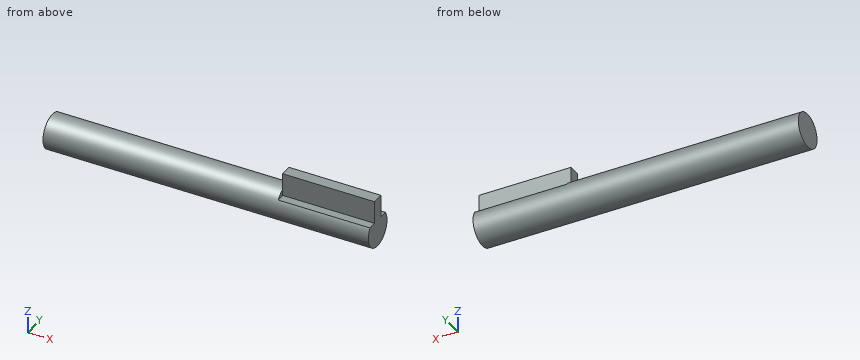
from build123d import *

# Parameters (mm, degrees)
F0_R     = 9.525
F1_DEPTH = 179.9844
F3_DEPTH = 50.8
F4_W     = 50.8
F4_H     = 6.35
F5_DEPTH = 12.7


with BuildPart() as f1:
    # F0 (on Right) → F1 (new body)
    with BuildSketch(Plane.YZ):
        Circle(F0_R)
    extrude(amount=-F1_DEPTH)

    # F2 (on face) → F3 (cut)
    with BuildSketch(Plane.YZ):
        with BuildLine():
            Line((-7.7629294276, 5.5192890577), (0, 5.5192890577))
            Line((0, 5.5192890577), (7.7629294276, 5.5192890577))
            ThreePointArc((7.7629294276, 5.5192890577), (0, 9.525), (-7.7629294276, 5.5192890577))
        make_face()
    extrude(amount=-F3_DEPTH, mode=Mode.SUBTRACT)

    # F4 (on face) → F5 (join)
    with BuildSketch(Plane.XY.offset(5.5192890577)):
        with Locations((-25.4, 0)):
            Rectangle(F4_W, F4_H)
    extrude(amount=F5_DEPTH)


solid = f1.part
Geometry check sheet. Reference: the model listing, model coordinates, mm. Give positions to 0.01 mm unless a question says otherwise; leave off trailing zeros. Loops run counter-clockwise (first coordinate to the right, second up) from the corner with the lowest first, then second, coordinate; pieces in that order, holes last. Notation, with made-up numbers: M 5.25,21.25 L 53.25,21.25 A24 cw 53.25,59.25 Z; hole C 30.25,58.25 d3. An arc over 180 degrees is marked long. Write each question's results on one line, items separated by ' | '.
1) Section check B-B, the plane z = 7. Record the boundary of the cut face in (x, y) (3 decimals), plus the area to 3 significant figures.
Answers follow:
outline: M -179.984,-6.46 L -50.8,-6.46 L -50.8,-3.175 L 0,-3.175 L 0,3.175 L -50.8,3.175 L -50.8,6.46 L -179.984,6.46 Z | area: 1,990 mm2
2) Section check C-C, the plane x = -38. Record the boundary of the cut face in (y, z) (3 decimals).
Answers follow:
outline: M -7.763,5.519 A9.525 ccw long 7.763,5.519 L 3.175,5.519 L 3.175,18.219 L -3.175,18.219 L -3.175,5.519 Z
3) Gauge pin test, flat ends, axial feed: pin 1 (1.7 mm diameter, centred on y = -5, z = 7, fed in from +X); pin 2 (6.5 mm diameter, centred on x = -26.5, z = 9, fed in from -Y) (3 decimals); pin 3 (1.4 mm diameter, centred on x = -33.5, y = -4.5, fed in from +Z). Record the tip position at first contact, or that the pin passes through.
Answers follow:
pin 1: x = -50.8 | pin 2: y = -3.175 | pin 3: z = 5.52
4) Section check A-A, the plane y = 0. Record the boundary of the cut face in (x, z) (3 decimals), plus the area to 3 significant figures.
Answers follow:
outline: M -179.984,-9.525 L 0,-9.525 L 0,18.219 L -50.8,18.219 L -50.8,9.525 L -179.984,9.525 Z | area: 3,870 mm2
5) Thickness scan on line 1 (Y direction, x = -14, z = 11.75) (3 decimals); line 2 (Z direction, x = -151, y = 0.5); line 3 (X direction, y = 3, z = 10.5). Record the ranges inside material, lowest first.
Answers follow:
line 1: -3.175 to 3.175 | line 2: -9.51 to 9.51 | line 3: -50.8 to 0
6) Section check D-D, the plane x = -101.5. Record the boundary of the cut face in (y, z) (3 decimals), plus the area to 3 significant figures.
Answers follow:
outline: C 0,0 d19.05 | area: 285 mm2
